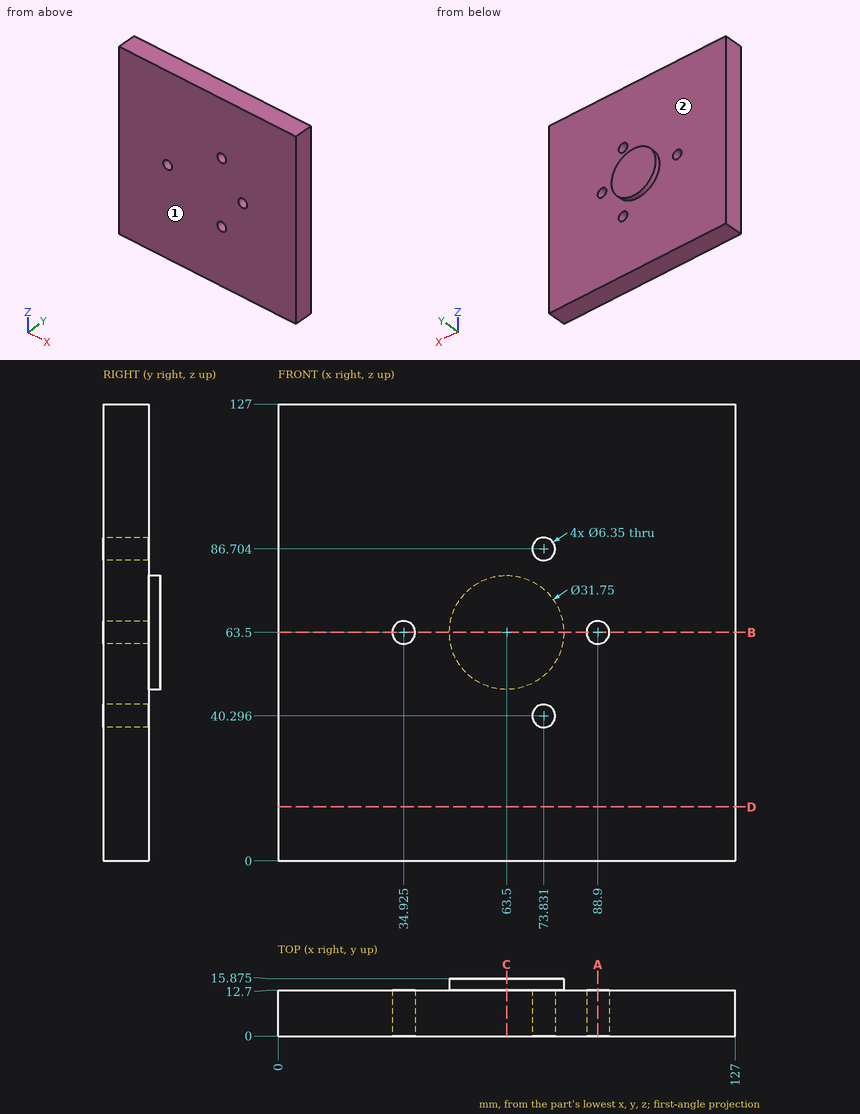
Part print with two shaded views. Sizes in mm from the minimum x, y, z corner. A direction names the side the tool comes from. Round coordinates to 2 decimals unless told otherwise and drop trailing zeros. Loops run counter-clockwise (first coordinate to the right, second up) from the corner with the lowest first, then second, coordinate; pieces in that order, holes last.
Item 1: Saw through at D-D (z = 15). List the corners of the cut face in (x, y), then the cut area to 3 significant figures.
Item 2: Which spindle directions (+Z, -Z, +X, -X, +Y, -Y) get a long thin tool onto all of the face, cutting with end or side? Do the marked faces 1 and 2. Say none if no direction does.
Item 3: Saw through at C-C (x = 63.5). List the corners of the cut face in (y, z) (3 decimals), then the cut area to 3 significant figures.
Item 4: Saw through at A-A (x = 88.9). List the corners of the cut face in (y, z) (3 decimals), then the cut area to 3 significant figures.
Item 5: Pin check, flat tip, straight feed: P1, Ø10, axis at x = 34.925, z = 63.5, coming from the +Y side. Stop position of the tip, or through.
Item 6: Saw through at B-B (z = 63.5). List the corners of the cut face in (x, y) (3 decimals).
Item 7: Drill centre lines: line 1 along X through (y, z) = (8, 63.5) (3 decimals); line 2 along Z through (x, y) = (88.9, 5.75) (3 decimals); line 3 along Y through (x, z) = (63.5, 88.5). Where is each one in solid material? Low to high.
Worked answers:
1. outline: (0, 0) - (127, 0) - (127, 12.7) - (0, 12.7) - close
1. area: 1,610 mm2
2. face 1: +Z, -Z, +X, -X, -Y
2. face 2: +Y
3. outline: (0, 0) - (12.7, 0) - (12.7, 47.625) - (15.875, 47.625) - (15.875, 79.375) - (12.7, 79.375) - (12.7, 127) - (0, 127) - close
3. area: 1,710 mm2
4. outline: (0, 0) - (12.7, 0) - (12.7, 60.325) - (0, 60.325) - close; (0, 66.675) - (12.7, 66.675) - (12.7, 127) - (0, 127) - close
4. area: 1,530 mm2
5. P1: stops at y = 12.7
6. outline: (0, 0) - (31.75, 0) - (31.75, 12.7) - (0, 12.7) - close; (38.1, 0) - (85.725, 0) - (85.725, 12.7) - (79.375, 12.7) - (79.375, 15.875) - (47.625, 15.875) - (47.625, 12.7) - (38.1, 12.7) - close; (92.075, 0) - (127, 0) - (127, 12.7) - (92.075, 12.7) - close
7. line 1: x = 0 to 31.75, 38.1 to 85.725, 92.075 to 127
7. line 2: z = 0 to 60.325, 66.675 to 127
7. line 3: y = 0 to 12.7
